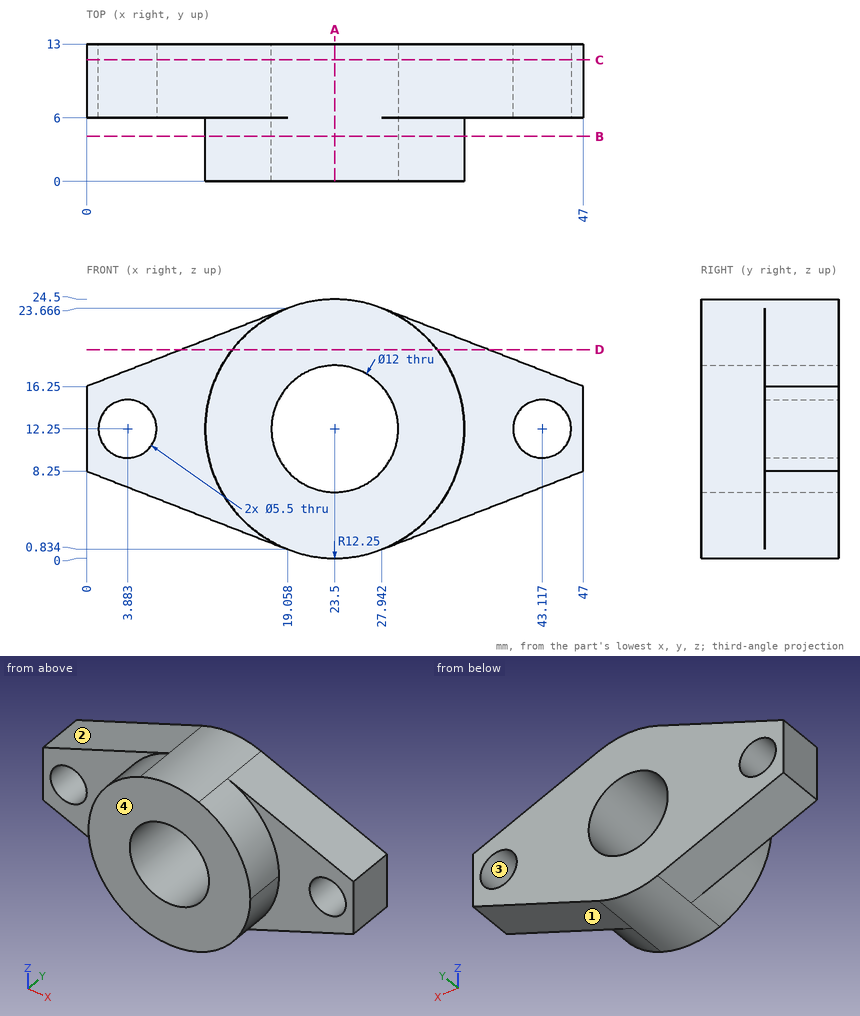
Here's the drawing with two shaded views (mm, measured from the low corner). I have some questions. Coordinates: 2 decimals unless noted, no trailing zeros. Write each loop counter-clockwise with the first axis right and the second up, starting at its lowest first coordinate (ties: lowest second). Pieces come first, ordered by that corner, then holes. Notation, with made-up numbers: M -38.5,-25.75 L -9.5,-25.75 A23 ccw -9.5,-1.75 Z; hole C 67.5,23.5 d3. An arc over 180 degrees is marked long. Write item = value, one per line. Start each with the question number.
Q1. If we section it at B-B, the plane y = 4.25: Write out the boundary of the cut face in (x, z).
Q2. If we section it at D-D, the plane z = 19.75: Write out the boundary of the cut face in (x, y) (1 decimal).
Q3. If we section it at C-C, the plane y = 11.5: Write out the boundary of the cut face in (x, z), then the cut area to 3 significant figures.
Q4. If we section it at A-A, the plane x = 23.5: Write out the boundary of the cut face in (y, z).
Q5. If I drill on L1, parallel to X at y = 9.25, z = 13; L2, parallel to X at y = 8.5, z = 14 (1 decimal); L3, parallel to Z at x = 23.5, y = 1, over which ranges is the centre line in solid material (lowest first)? Write a range as [from, to].
Q6. I'm going to push flat-ended pins straight in: pin 1 (1 mm diameter, centred on y = 3.5, z = 20.5, fed in from -X); pin 2 (5.5 mm diameter, centred on x = 41, z = 10.5, fed in from -Y); pin 3 (4 mm diameter, centred on x = 35, y = 8.5, fed in from +Z). Where does each tip first touch, or does it pass through?
Q7. Thinking about a two-plate mould opening in X: for the marked faces 1, 2, 3 and 4, which applies, released by +X, released by -X, zero draft, split by the parting line, or undercut?
Check sheet entries:
q1.outline = M 19.06,23.67 A12.25 ccw 27.94,0.83 A12.25 ccw 35.75,12.25 A12.25 ccw 27.94,23.67 A12.25 ccw Z; hole C 23.5,12.25 d12
q2.outline = M 9,6 L 13.8,6 L 13.8,0 L 33.2,0 L 33.2,6 L 38,6 L 38,13 L 9,13 Z
q3.outline = M 0,8.25 L 19.06,0.83 A12.25 ccw 27.94,0.83 L 47,8.25 L 47,16.25 L 27.94,23.67 A12.25 ccw 19.06,23.67 L 0,16.25 Z; hole C 3.88,12.25 d5.5; hole C 23.5,12.25 d12; hole C 43.12,12.25 d5.5
q3.area = 640 mm²
q4.outline = M 0,0 L 13,0 L 13,6.25 L 0,6.25 Z; M 0,18.25 L 13,18.25 L 13,24.5 L 0,24.5 Z
q5.L1 = [0, 1.24], [6.53, 17.55], [29.45, 40.47], [45.76, 47]
q5.L2 = [0, 1.8], [6, 17.8], [29.2, 41], [45.2, 47]
q5.L3 = [0, 6.25], [18.25, 24.5]
q6.pin_1 = 14.01
q6.pin_2 = 6
q6.pin_3 = 21.7
q7.face_1 = released by +X
q7.face_2 = released by -X
q7.face_3 = undercut
q7.face_4 = zero draft
